```python
from build123d import *

# Parameters (mm, degrees)
SKETCH1_W           = 17
SKETCH1_H           = 17
BOSS_EXTRUDE1_DEPTH = 1
SKETCH2_W           = 14
SKETCH2_H           = 14
SKETCH2_W_2         = 10
SKETCH2_H_2         = 10
BOSS_EXTRUDE2_DEPTH = 4
FILLET1_R           = 2


with BuildPart() as part:
    # Sketch1 → Boss-Extrude1 (new body)
    with BuildSketch(Plane(origin=(0, 0, 0), x_dir=(1, 0, 0), z_dir=(0, 1, 0))):
        Rectangle(SKETCH1_W, SKETCH1_H)
    extrude(amount=BOSS_EXTRUDE1_DEPTH)

    # Sketch2 → Boss-Extrude2 (add)
    with BuildSketch(Plane(origin=(0, 1, 0), x_dir=(1, 0, 0), z_dir=(0, 1, 0))):
        Rectangle(SKETCH2_W, SKETCH2_H)
        Rectangle(SKETCH2_W_2, SKETCH2_H_2, mode=Mode.SUBTRACT)
    extrude(amount=BOSS_EXTRUDE2_DEPTH)

    # Fillet1
    fillet1_edges = [part.edges().sort_by_distance(p)[0] for p in [
        (7, 3, 7),
        (7, 3, -7),
        (-7, 3, -7),
        (-7, 3, 7),
        (-5, 3, -5),
        (-5, 3, 5),
        (5, 3, 5),
        (5, 3, -5),
    ]]
    fillet(fillet1_edges, radius=FILLET1_R)


solid = part.part
```
Verification items for the finished model (mm, model axes). A direction names the side the tool comes from. Round coordinates to 2 decimals unless told otherwise and drop trailing zeros. Order: outer loops, then holes, each group sorted by start corner. A loop starts at its lowest first (then second) coordinate and runs counter-clockwise, first axis right, second up.
1) Depth check by flat-ended pin: pin 1 (2 mm diameter, centred on x = 0, y = 3.5, fed in from +Z); pin 2 (3 mm diameter, centred on x = 0, y = 3.5, fed in from -Z); pin 3 (1.2 mm diameter, centred on y = 3, z = -0.5, fed in from -X). Enter the tip coordinate at first touch or a pass-through.
Geometry says:
pin 1: stops at z = 7
pin 2: stops at z = -7
pin 3: stops at x = -7
2) Cross-section at B-B, the plane x = -0.5. Record the cut outline in (y, z), plus the area to 3 significant figures.
Geometry says:
outline: (0, -8.5) - (1, -8.5) - (1, -7) - (5, -7) - (5, -5) - (1, -5) - (1, 5) - (5, 5) - (5, 7) - (1, 7) - (1, 8.5) - (0, 8.5) - close
area: 33.0 mm2
3) Tool access check on faces 1 (the flat face through (-7, 3, 0)), 2 (the cylindrical face through (4.4, 3.03, 4.43)), 3 (the cylindrical face through (-6.4, 3.03, 6.43)), 4 (the cylindrical face through (6.4, 3.03, 6.43)), 5 (the cylindrical face through (6.43, 3.03, -6.4)). Record the directions out of +Z, -Z, +X, -X, +Y, -Y that give a thin tool (end or side, any length) a straight path to the whole face; none if there is none.
Geometry says:
face 1: +Z, -Z, -X, +Y
face 2: +Y
face 3: +Z, -X, +Y
face 4: +Z, +X, +Y
face 5: -Z, +X, +Y
4) Draft check along X on faces 6 (the flat face through (5, 3, 0)), 7 (the cylindrical face through (-4.4, 3.03, -4.43)), 8 (the flat face through (8.5, 0.5, 0.1)), 9 (the flat face through (0, 0, 0)). Enter one of: +X half, -X half, draft (parallel to the pull), parting line (faces both ways), or undercut.
Geometry says:
face 6: undercut
face 7: undercut
face 8: +X half
face 9: draft
5) Material ranges on line 1 (X direction, y = 3.6, z = 2.5); line 2 (Y direction, x = -7.5, z = 1.75), recorded low to high.
Geometry says:
line 1: x = -7 to -5, 5 to 7
line 2: y = 0 to 1
6) Cross-section at C-C, the plane z = -1.75. Record the cut outline in (x, y).
Geometry says:
outline: (-8.5, 0) - (8.5, 0) - (8.5, 1) - (7, 1) - (7, 5) - (5, 5) - (5, 1) - (-5, 1) - (-5, 5) - (-7, 5) - (-7, 1) - (-8.5, 1) - close
7) Cross-section at A-A, the plane y = 3.35. Record the cut outline in (x, z), plus the area to 3 significant figures.
Geometry says:
outline: (-7, -5) arc R2 ccw to (-5, -7) - (5, -7) arc R2 ccw to (7, -5) - (7, 5) arc R2 ccw to (5, 7) - (-5, 7) arc R2 ccw to (-7, 5) - close; hole (-5, -3) arc R2 ccw to (-3, -5) - (3, -5) arc R2 ccw to (5, -3) - (5, 3) arc R2 ccw to (3, 5) - (-3, 5) arc R2 ccw to (-5, 3) - close
area: 96.0 mm2
8) Cross-section at D-D, the plane x = 5.5. Record the cut outline in (y, z).
Geometry says:
outline: (0, -8.5) - (1, -8.5) - (1, -6.94) - (5, -6.94) - (5, 6.94) - (1, 6.94) - (1, 8.5) - (0, 8.5) - close
